from build123d import *

# Parameters (mm, degrees)
SKETCH1_W           = 38.1
SKETCH1_H           = 101.6
BOSS_EXTRUDE1_DEPTH = 6.35
FILLET1_R           = 5
FILLET2_R           = 5
FILLET3_R           = 5
FILLET4_R           = 5
CUT_EXTRUDE1_REACH  = 180.93
SKETCH2_R           = 4.445


with BuildPart() as part:
    # Sketch1 → Boss-Extrude1 (new body)
    with BuildSketch(Plane.XY):
        with Locations((0, -127)):
            Rectangle(SKETCH1_W, SKETCH1_H)
        with BuildLine():
            Line((-12.222, -110.928), (-12.222, -135.128))
            ThreePointArc((-12.222, -135.128), (-11.501276628, -139.562051447), (-9.413312538, -143.539570822))
            Line((-9.413312538, -143.539570822), (-9.95027795, -143.990138361))
            ThreePointArc((-9.95027795, -143.990138361), (-9.482853323, -144.576977852), (-8.986096678, -145.139204858))
            Line((-8.986096678, -145.139204858), (-8.44913124, -144.688637356))
            ThreePointArc((-8.44913124, -144.688637356), (1.777999803, -149.128000002), (12.005130971, -144.688637644))
            Line((12.005130971, -144.688637644), (12.542096526, -145.139205022))
            ThreePointArc((12.542096526, -145.139205022), (13.038853251, -144.576977937), (13.506277951, -143.99013836))
            Line((13.506277951, -143.99013836), (12.969312655, -143.539570964))
            ThreePointArc((12.969312655, -143.539570964), (15.057276792, -139.562051525), (15.77800018, -135.128))
            Line((15.77800018, -135.128), (15.77800018, -110.928))
            ThreePointArc((15.77800018, -110.928), (15.485106961, -110.220893219), (14.77800018, -109.928))
            Line((14.77800018, -109.928), (-11.222, -109.928))
            ThreePointArc((-11.222, -109.928), (-11.929106781, -110.220893219), (-12.222, -110.928))
        make_face(mode=Mode.SUBTRACT)
    extrude(amount=BOSS_EXTRUDE1_DEPTH)

    # Fillet1
    fillet1_edges = [part.edges().sort_by_distance(p)[0] for p in [
        (-19.05, -76.2, 3.175),
    ]]
    fillet(fillet1_edges, radius=FILLET1_R)

    # Fillet2
    fillet2_edges = [part.edges().sort_by_distance(p)[0] for p in [
        (19.05, -76.2, 3.175),
    ]]
    fillet(fillet2_edges, radius=FILLET2_R)

    # Fillet3
    fillet3_edges = [part.edges().sort_by_distance(p)[0] for p in [
        (19.05, -177.8, 3.175),
    ]]
    fillet(fillet3_edges, radius=FILLET3_R)

    # Fillet4
    fillet4_edges = [part.edges().sort_by_distance(p)[0] for p in [
        (-19.05, -177.8, 3.175),
    ]]
    fillet(fillet4_edges, radius=FILLET4_R)

    # Sketch2 → Cut-Extrude1 (cut, up to next)
    with BuildSketch(Plane.XY.offset(6.35), mode=Mode.PRIVATE) as cut_extrude1_sk1:
        with Locations((0, -93.234389415)):
            Circle(SKETCH2_R)
    cut_extrude1_tool1 = extrude(cut_extrude1_sk1.sketch, amount=-CUT_EXTRUDE1_REACH, mode=Mode.PRIVATE) & part.part
    # Sketch2 → Cut-Extrude1 (cut, up to next)
    with BuildSketch(Plane.XY.offset(6.35), mode=Mode.PRIVATE) as cut_extrude1_sk2:
        with Locations((0, -165.643685175)):
            Circle(SKETCH2_R)
    cut_extrude1_tool2 = extrude(cut_extrude1_sk2.sketch, amount=-CUT_EXTRUDE1_REACH, mode=Mode.PRIVATE) & part.part
    add(cut_extrude1_tool1.solids().sort_by_distance((0, -93.234389, 6.35))[0], mode=Mode.SUBTRACT)
    add(cut_extrude1_tool2.solids().sort_by_distance((0, -165.643685, 6.35))[0], mode=Mode.SUBTRACT)


solid = part.part
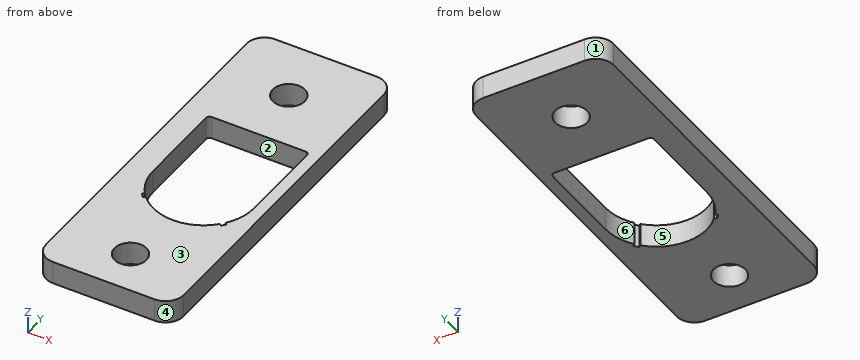
Work out the finished part from the listing and answer in its coordinate system (mm). Face numbers are marked on the shaded views. A direction names the side the tool comes from. Give positions to 0.01 mm unless a question says otherwise; leave off trailing zeros. Loops run counter-clockwise (first coordinate to the right, second up) from the corner with the lowest first, then second, coordinate; pieces in that order, holes last. Notation, with made-up numbers: (89, -20) -> (115, -20) arc R29 cw to (115, 11) -> close; hole circle Ø10 at (75.5, 12). An arc over 180 degrees is marked (long way). Use a Markdown table: item, result. Add a question column.
1) Which of the six approach directions +Z, -Z, +X, -X, +Y, -Y give full straight-line access (tool end or side, diameter ignored) to the marked faces 1 and 2?
2) The part is cut by section A-A, the plane y = -136. Determine the outline of the cut face in (x, z).
3) Consider line 1 along X through (y, z) = (-112.5, 2.25); line 2 along Y through (x, z) = (-9, 6); line 3 along Y through (x, z) = (0, 4.5). Determine where each line is inside the solid, lowest interval first.
4) The part is cut by section B-B, the plane x = 2. Determine the outline of the cut face in (y, z).
5) For a pull along X with two mould halves and no side action, classify the marked faces 3, 4, 5 and 6 as +X half, -X half, draft (parallel to the pull), parting line (faces both ways), or undercut.
6) The part is cut by section D-D, the plane x = -6.5. Determine the outline of the cut face in (y, z).
7) The part is cut by section C-C, the plane z = 3.5. Determine the outline of the cut face in (x, y) (3 decimals).
Reported:
| question | item | result |
|---|---|---|
| 1 | face 1 | +Z, -Z, -X, +Y |
| 1 | face 2 | +Z, -Z |
| 2 | outline | (-19.05, 0) -> (-12.19, 0) -> (-12.19, 6.35) -> (-19.05, 6.35) -> close; (15.75, 0) -> (19.05, 0) -> (19.05, 6.35) -> (15.75, 6.35) -> close |
| 3 | line 1 | x = -19.05 to -12.22, 15.78 to 19.05 |
| 3 | line 2 | y = -177.8 to -145.12, -109.93 to -76.2 |
| 3 | line 3 | y = -177.8 to -170.09, -161.2 to -149.01, -109.93 to -97.68, -88.79 to -76.2 |
| 4 | outline | (-177.8, 0) -> (-169.61, 0) -> (-169.61, 6.35) -> (-177.8, 6.35) -> close; (-161.67, 0) -> (-149.13, 0) -> (-149.13, 6.35) -> (-161.67, 6.35) -> close; (-109.93, 0) -> (-97.2, 0) -> (-97.2, 6.35) -> (-109.93, 6.35) -> close; (-89.26, 0) -> (-76.2, 0) -> (-76.2, 6.35) -> (-89.26, 6.35) -> close |
| 5 | face 3 | draft |
| 5 | face 4 | +X half |
| 5 | face 5 | undercut |
| 5 | face 6 | undercut |
| 6 | outline | (-177.8, 0) -> (-146.42, 0) -> (-146.42, 6.35) -> (-177.8, 6.35) -> close; (-109.93, 0) -> (-76.2, 0) -> (-76.2, 6.35) -> (-109.93, 6.35) -> close |
| 7 | outline | (-19.05, -172.8) arc R5 ccw to (-14.05, -177.8) -> (14.05, -177.8) arc R5 ccw to (19.05, -172.8) -> (19.05, -81.2) arc R5 ccw to (14.05, -76.2) -> (-14.05, -76.2) arc R5 ccw to (-19.05, -81.2) -> close; hole (-12.222, -135.128) arc R14 ccw to (-9.413, -143.54) -> (-9.95, -143.99) arc R14.7 ccw to (-8.986, -145.139) -> (-8.449, -144.689) arc R14 ccw to (12.005, -144.689) -> (12.542, -145.139) arc R14.7 ccw to (13.506, -143.99) -> (12.969, -143.54) arc R14 ccw to (15.778, -135.128) -> (15.778, -110.928) arc R1 ccw to (14.778, -109.928) -> (-11.222, -109.928) arc R1 ccw to (-12.222, -110.928) -> close; hole circle Ø8.89 at (0, -165.644); hole circle Ø8.89 at (0, -93.234) |
